Source: CAD feature listing. Evaluate the final solid. Frame: model axes, mm. Give positions to 0.01 mm unless a question says otherwise; leave off trailing zeros.
```python
from build123d import *

# Parameters (mm, degrees)
ESBO_O1_W                = 1500
ESBO_O1_H                = 1800
RESSALTO_EXTRUS_O1_DEPTH = 10
ESBO_O2_R                = 40
CORTE_EXTRUS_O1_DEPTH    = 11
FURO_COM_FOLGA_DE_M61_D  = 6.6


with BuildPart() as part:
    # Esboço1 → Ressalto-extrusão1 (new body)
    with BuildSketch(Plane.XY):
        Rectangle(ESBO_O1_W, ESBO_O1_H)
    extrude(amount=RESSALTO_EXTRUS_O1_DEPTH)

    # Esboço2 → Corte-extrusão1 (cut, through all)
    with BuildSketch(Plane.XY.offset(10)):
        with Locations((350, 0)):
            Circle(ESBO_O2_R)
    extrude(amount=-CORTE_EXTRUS_O1_DEPTH, mode=Mode.SUBTRACT)

    # Furo com folga de M61 (through all)
    with Locations(Plane(origin=(350, 0, 16), x_dir=(0, 1, 0), z_dir=(0, 0, 1))):
        with Locations((0, 1038.39252282), (355.151159483, 975.769791173), (667.46584766, 795.454821883), (-355.151159483, 975.769791173), (-667.46584766, 795.454821883)):
            Hole(FURO_COM_FOLGA_DE_M61_D / 2)


solid = part.part
```
(1) First-contact query: pin 1 (7.5 mm diameter, centred on x = -688.39, y = 0, fed in from -Z); pin 2 (5.5 mm diameter, centred on x = -625.77, y = 355.15, fed in from -Z). Flat tips, straight axial feed; report the tip coordinate or a pass-through.
A:
pin 1: stops at z = 0
pin 2: passes through
(2) Mould query, pull axis X, two halves, no side actions, for faces 1 (the cylindrical face through (310.04, 1.76, 5.07)), 2 (the flat face through (-10, 13, 0)). Classes: pulls with the +X half, pulls with the -X half, needs draft (parallel to the pull), parting line crosses it, or undercut.
A:
face 1: undercut
face 2: needs draft
(3) Ray query, line 1 along Y through (x, z) = (350, 5); line 2 along Y through (x, z) = (321, 3); line 3 along X through (y, z) = (25.5, 7.75). Return the intervals inside material, ascending.
A:
line 1: y = -900 to -40, 40 to 900
line 2: y = -900 to -27.55, 27.55 to 900
line 3: x = -750 to 319.18, 380.82 to 750
